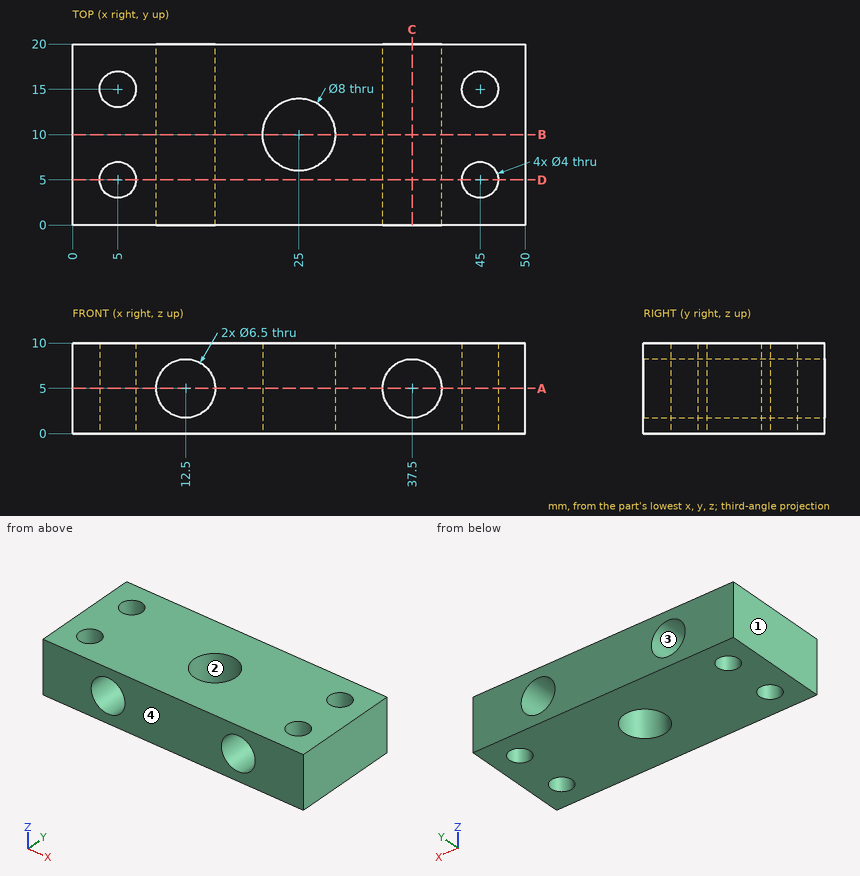
For this review, use the dimensioned drawing (mm, ordinates from the lowest corner) and the shaded views. Round coordinates to 2 decimals unless told otherwise and drop trailing zeros. Loops run counter-clockwise (first coordinate to the right, second up) from the corner with the lowest first, then second, coordinate; pieces in that order, holes last. Notation, with made-up numbers: M 12,43 L 60,43 A25 cw 60,74 Z; hole C -15.75,-13.75 d3. An arc over 180 degrees is marked long. Answer as a JSON object with one key per item and string values.
(1) Draft analysis for pull direction X (two halves, no side actions). For the marked faces 1, 2, 3 and 4, state which applies: released by +X, released by -X, zero draft, split by the parting line, or undercut.
Resolved:
{"face 1": "released by -X", "face 2": "undercut", "face 3": "undercut", "face 4": "zero draft"}
(2) Take a section at A-A on z = 5. Give the boundary of the cut face in (x, y), and give its area (3 significant figures).
Resolved:
{"outline": "M 0,0 L 9.25,0 L 9.25,20 L 0,20 Z; M 15.75,0 L 34.25,0 L 34.25,20 L 15.75,20 Z; M 40.75,0 L 50,0 L 50,20 L 40.75,20 Z; hole C 5,5 d4; hole C 5,15 d4; hole C 25,10 d8; hole C 45,5 d4; hole C 45,15 d4", "area": "639 mm²"}
(3) Take a section at B-B on y = 10. Give the boundary of the cut face in (x, z).
Resolved:
{"outline": "M 0,0 L 21,0 L 21,10 L 0,10 Z; M 29,0 L 50,0 L 50,10 L 29,10 Z; hole C 12.5,5 d6.5; hole C 37.5,5 d6.5"}
(4) Clearance check with a flat-ended pin moving along its axis: P1, Ø6, axis at x = 12.5, z = 5, coming from the -Y side. State where the tip first meets the part, or that it passes through.
Resolved:
{"P1": "through"}
(5) Take a section at D-D on y = 5. Give the boundary of the cut face in (x, z).
Resolved:
{"outline": "M 0,0 L 3,0 L 3,10 L 0,10 Z; M 7,0 L 43,0 L 43,10 L 7,10 Z; M 47,0 L 50,0 L 50,10 L 47,10 Z; hole C 12.5,5 d6.5; hole C 37.5,5 d6.5"}
(6) Take a section at C-C on x = 37.5. Give the boundary of the cut face in (y, z).
Resolved:
{"outline": "M 0,0 L 20,0 L 20,1.75 L 0,1.75 Z; M 0,8.25 L 20,8.25 L 20,10 L 0,10 Z"}
(7) To check wall thickness, follow line 1 along X through (y, z) = (10, 4.75); line 2 along Y through (x, z) = (45, 6.25); line 3 along X through (y, z) = (13.5, 1). State the ranges of each line that lie inside material, in increasing order.
Resolved:
{"line 1": "0 to 9.26, 15.74 to 21, 29 to 34.26, 40.74 to 50", "line 2": "0 to 3, 7 to 13, 17 to 20", "line 3": "0 to 3.68, 6.32 to 23.06, 26.94 to 43.68, 46.32 to 50"}
